Autodesk Inventor part; units mm, degrees
ref_plane "YZ Plane" through (0, 0, 0) normal (1, 0, 0) x (0, 1, 0)
ref_plane "XZ Plane" through (0, 0, 0) normal (0, 1, 0) x (-1, 0, 0)
ref_plane "XY Plane" through (0, 0, 0) normal (0, 0, 1) x (1, 0, 0)
sketch "Sketch1" plane through (0, 0, 0) normal (1, 0, 0) x (0, 1, 0)
  line L0 (-129, 130) -> (129, 130)
  line L1 (129, 130) -> (129, -130)
  line L2 (129, -130) -> (-129, -130)
  line L3 (-129, -130) -> (-129, 130)
  line L4 (-129, 130) -> (129, -130) construction
  line L5 (129, 130) -> (-129, -130) construction
  point P0 (0, 0)
  dimension "d0" = 258
  dimension "d1" = 260
extrude "Extrusion1" add sketch "Sketch1" along normal mid plane 5
sketch "Sketch3" plane through (-2.5, 0, 0) normal (-1, 0, 0) x (0, 0, 1)
  circle A0 centre (100.5, -99.5) radius 16.7557 construction
  line L0 (130, -129) -> (130, 129) construction
  line L1 (-130, -129) -> (130, -129) construction
  circle A1 centre (100.5, -99.5) radius 14
  point P0 (0, 0)
  dimension "d12" = 29.5
  dimension "d13" = 29.5
  dimension "d14" = 28
extrude "Extrusion3" cut sketch "Sketch3" against normal blind 5
sketch "Sketch4" plane through (-2.5, 0, 0) normal (-1, 0, 0) x (0, 0, 1)
  circle A0 centre (107.5, 3.5) radius 12.5 construction
  line L0 (130, -129) -> (130, 129) construction
  line L1 (-130, -129) -> (130, -129) construction
  circle A1 centre (107.5, 3.5) radius 8
  circle A2 centre (62.5, 3.5) radius 12.5 construction
  circle A3 centre (62.5, 3.5) radius 8
  point P0 (0, 0)
  dimension "d17" = 25
  dimension "d18" = 22.5
  dimension "d19" = 132.5
  dimension "d20" = 16
  dimension "d21" = 25
  dimension "d22" = 45
  dimension "d23" = 16
  dimension "d24" = 132.5
extrude "Extrusion4" cut sketch "Sketch4" against normal blind 5
equation "\"d0\" = boxh"
equation "\"d1\" = boxl + 2 * pvct"
equation "\"d2\" = pvct"
equation "\"d14\" = airininner"
equation "\"d15\" = pvct"
equation "\"d17\" = diapowerouter"
equation "\"d20\" = diapower"
equation "\"d21\" = diapowerouter"
equation "\"d23\" = diapower"
equation "\"d25\" = pvct"
equation "\"solhole\" = 3"
equation "\"solholespacing\" = 16"
equation "\"ssolw\" = 63"
equation "\"bsoll\" = 126"
equation "\"bsolw\" = 91"
equation "\"bsolh\" = 126"
equation "\"tapl\" = 31"
equation "\"tl\" = 32"
equation "\"eloboww\" = 25"
equation "\"pvct\" = 5"
equation "\"boxh\" = 258"
equation "\"supporth\" = 15"
equation "\"play\" = 0.5"
equation "\"pcbh\" = 46"
equation "\"pcbw\" = 76"
equation "\"pcbl\" = 86"
equation "\"arl\" = 102"
equation "\"arw\" = 54"
equation "\"psuh\" = 85"
equation "\"screenl\" = 115"
equation "\"screenw\" = 197"
equation "\"seph\" = 105"
equation "\"diapowerouter\" = 25"
equation "\"dialoadouter\" = 25"
equation "\"distpumps\" = 75"
equation "\"diaetapeouter\" = 36"
equation "\"diaphouter\" = 48"
equation "\"distbubblewater\" = 82"
equation "\"diaload\" = 16"
equation "\"diaetape\" = 25"
equation "\"diaph\" = 32"
equation "\"diapower\" = 16"
equation "\"pumpouter\" = 25"
equation "\"airoutinner\" = 28"
equation "\"airoutouter\" = 39"
equation "\"waterouter\" = 39"
equation "\"waterinner\" = 28"
equation "\"pumpinner\" = 16"
equation "\"airininner\" = 28"
equation "\"airinouter\" = 39"
properties part number "sb_side" material "PVC-Piping"
Check sheet for the modelled part. Datum: model origin and axes. Units: mm. Give positions to 0.01 mm unless a question says otherwise; leave off trailing zeros. Loops run counter-clockwise (first coordinate to the right, second up) from the corner with the lowest first, then second, coordinate; pieces in that order, holes last. Notation, with made-up numbers: M 69.5,75 L 118.5,75 A17 ccw 118.5,102 Z; hole C -28,77.5 d4. An arc over 180 degrees is marked long. Answer in a Markdown table with one row per item.
1) Cross-section at B-B (x = -1.1). Enter the section's corners in (y, z), plus the area to 3 significant figures.
Solutions:
| item | result |
|---|---|
| outline | M -129,-130 L 129,-130 L 129,130 L -129,130 Z; hole C -99.5,100.5 d28; hole C 3.5,62.5 d16; hole C 3.5,107.5 d16 |
| area | 66,100 mm^2 |
2) Thickness scan on line 1 (Y direction, x = -0.15, z = 110); line 2 (Y direction, x = -0.25, z = 62.5); line 3 (Y direction, x = 0.7, z = 100.5). Record the ranges inside material, lowest first.
Solutions:
| item | result |
|---|---|
| line 1 | y = -129 to -109.78, -89.22 to -4.1, 11.1 to 129 |
| line 2 | y = -129 to -4.5, 11.5 to 129 |
| line 3 | y = -129 to -113.5, -85.5 to -0.37, 7.37 to 129 |
3) Cross-section at C-C (z = 62.5). Enter the section's corners in (x, y), plus the area to 3 significant figures.
Solutions:
| item | result |
|---|---|
| outline | M -2.5,-129 L 2.5,-129 L 2.5,-4.5 L -2.5,-4.5 Z; M -2.5,11.5 L 2.5,11.5 L 2.5,129 L -2.5,129 Z |
| area | 1,210 mm^2 |
4) Cross-section at D-D (z = 107.5). Enter the section's corners in (x, y), plus the area to 3 significant figures.
Solutions:
| item | result |
|---|---|
| outline | M -2.5,-129 L 2.5,-129 L 2.5,-111.62 L -2.5,-111.62 Z; M -2.5,-87.38 L 2.5,-87.38 L 2.5,-4.5 L -2.5,-4.5 Z; M -2.5,11.5 L 2.5,11.5 L 2.5,129 L -2.5,129 Z |
| area | 1,090 mm^2 |
5) Cross-section at A-A (y = -99.5). Enter the section's corners in (x, z), plus the area to 3 significant figures.
Solutions:
| item | result |
|---|---|
| outline | M -2.5,-130 L 2.5,-130 L 2.5,86.5 L -2.5,86.5 Z; M -2.5,114.5 L 2.5,114.5 L 2.5,130 L -2.5,130 Z |
| area | 1,160 mm^2 |
6) Depth check by flat-ended pin: pin 1 (14.5 mm diameter, centred on y = 3.5, z = 62.5, fed in from -X). Enter the tip coordinate at first touch or a pass-through.
Solutions:
| item | result |
|---|---|
| pin 1 | passes through |
7) Mould release check, pull along Z, two halves, no side actions. Record for faces 1 (the face through (-2.5, -2, 2)), 2 (the face through (-0.035, -87.695, 108.026)): released by +Z, released by -Z, zero draft, split by the parting line, or undercut.
Solutions:
| item | result |
|---|---|
| face 1 | zero draft |
| face 2 | undercut |
